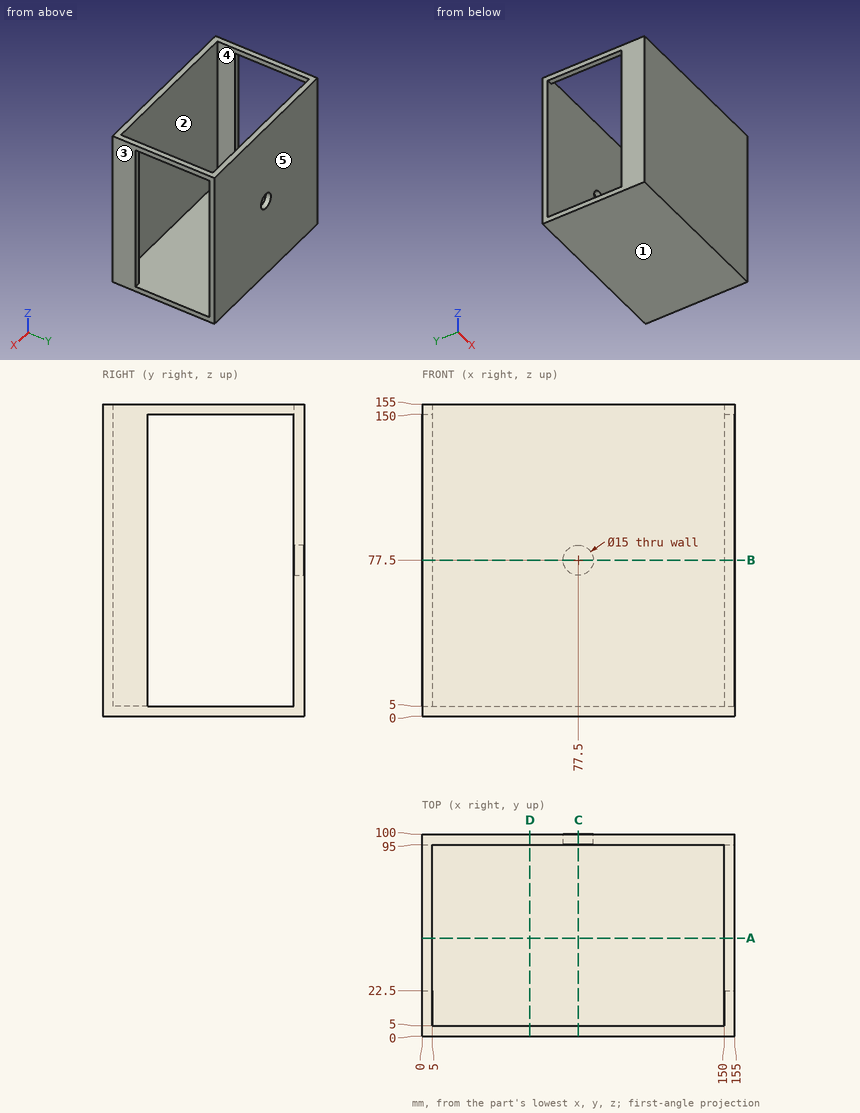
Can you work these out from the drawing? Everything is in mm from the part's minimum corner. A direction names the side the tool comes from. Round coordinates to 2 decimals unless told otherwise and drop trailing zeros. Write each loop counter-clockwise with the first axis right and the second up, starting at its lowest first coordinate (ties: lowest second). Pieces come first, ordered by that corner, then holes.
1. Will this pin go through, and if not, where does the flat tip stop? pin 1 Ø8 at (x, y) = (106.5, 89) entering from +Z.
2. Suppose I cut it at D-D (x = 53.5). List the corners of the cut face in (y, z) for me, and give its area (3 significant figures).
3. I need wall thicknesses on L1, parallel to Z at x = 77, y = 96; L2, parallel to Y at x = 45.5, z = 50; L3, parallel to X at y = 17, z = 27. Which ranges of each line are inside material? Lowest first, please.
4. Suppose I cut it at C-C (x = 77.5). List the corners of the cut face in (y, z) for me.
5. Suppose I cut it at B-B (z = 77.5). List the corners of the cut face in (x, y) for me.
6. If we mould it in two halves opening along X, with no side actions, what happens to the marked faces 3, 4 and 5? For each: released by +X, released by -X, zero draft, split by the parting line, or undercut.
7. For the marked faces 1 and 2, which set-ups out of +Z, -Z, +X, -X, +Y, -Y let a thin tool reach every point of the face, with its end or its side?
8. Suppose I cut it at A-A (y = 48.5). List the corners of the cut face in (x, z) for me.
Answer sheet:
1. pin 1: stops at z = 5
2. outline: (0, 0) - (100, 0) - (100, 155) - (95, 155) - (95, 5) - (5, 5) - (5, 155) - (0, 155) - close
2. area: 2,000 mm2
3. L1: z = 0 to 70.02, 84.98 to 155
3. L2: y = 0 to 5, 95 to 100
3. L3: x = 0 to 5, 150 to 155
4. outline: (0, 0) - (100, 0) - (100, 70) - (95, 70) - (95, 5) - (5, 5) - (5, 155) - (0, 155) - close; (95, 85) - (100, 85) - (100, 155) - (95, 155) - close
5. outline: (0, 0) - (155, 0) - (155, 22.5) - (150, 22.5) - (150, 5) - (5, 5) - (5, 22.5) - (0, 22.5) - close; (0, 95) - (70, 95) - (70, 100) - (0, 100) - close; (85, 95) - (155, 95) - (155, 100) - (85, 100) - close
6. face 3: released by +X
6. face 4: undercut
6. face 5: zero draft
7. face 1: -Z, +X, -X, +Y, -Y
7. face 2: +Z
8. outline: (0, 0) - (155, 0) - (155, 5) - (0, 5) - close; (0, 150) - (5, 150) - (5, 155) - (0, 155) - close; (150, 150) - (155, 150) - (155, 155) - (150, 155) - close
